Can you work these out from the model? Positions are in its coordinate system, mm. Round coordinates to 2 decimals unless told otherwise and drop trailing zeros. Loops run counter-clockwise (first coordinate to the right, second up) from the corner with the lowest first, then second, coordinate; pieces in that order, holes last.
(1) I want a section at B-B on x = 148.75. Write out the boundary of the cut face in (y, z), plus the area to 3 significant figures.
(2) I want a section at A-A on z = 51. Write out the boundary of the cut face in (x, y).
(3) Thinking about a two-plate mould opening in Z: for faces 1 (the face through (89, 0, 59)), 2 (the face through (176.99, 0.74, 17.85)), 3 (the face through (89.34, 0.76, 32.24)), 4 (the face through (176.99, 0.74, 102.15)), which applies, released by +Z, released by -Z, zero draft, split by the parting line, or undercut?
(4) I want a section at C-C on y = 1.2. Give the number of separate pieces and of enclosed holes in the cut face, plus the area to 3 significant figures.
(5) If I drill on line 1 along X through (y, z) = (0.3, 60); line 2 along Z through (x, y) = (148.75, 0.65); line 3 along X through (y, z) = (0.35, 31.25), over which ranges is the centre line in solid material (lowest first)?
(6) I want a section at D-D on x = 129. Write out the boundary of the cut face in (y, z).
from build123d import *

# Parameters (mm, degrees)
SKETCH1_W           = 180
SKETCH1_H           = 120
BOSS_EXTRUDE1_DEPTH = 1.5
SKETCH2_R           = 2.15
CUT_EXTRUDE1_DEPTH  = 217.33827678
SKETCH3_W           = 180
SKETCH3_H           = 15
CUT_EXTRUDE2_DEPTH  = 217.33827678
FILLET1_R           = 10


with BuildPart() as part:
    # Sketch1 → Boss-Extrude1 (new body)
    with BuildSketch(Plane(origin=(0, 0, 0), x_dir=(1, 0, 0), z_dir=(0, 1, 0))):
        with Locations((90, -60)):
            Rectangle(SKETCH1_W, SKETCH1_H)
    extrude(amount=BOSS_EXTRUDE1_DEPTH)

    # Sketch2 → Cut-Extrude1 (cut, through all)
    with BuildSketch(Plane(origin=(0, 1.5, 0), x_dir=(1, 0, 0), z_dir=(0, 1, 0))):
        with Locations(Location((120, -51, 0), (0, 0, 270))):
            Circle(SKETCH2_R)
        with Locations(Location((120, -69, 0), (0, 0, 270))):
            Circle(SKETCH2_R)
        with Locations(Location((129, -60, 0), (0, 0, 270))):
            Circle(SKETCH2_R)
        with Locations(Location((111, -60, 0), (0, 0, 270))):
            Circle(SKETCH2_R)
        with Locations(Location((78, -51, 0), (0, 0, 270))):
            Circle(SKETCH2_R)
        with Locations(Location((62, -51, 0), (0, 0, 270))):
            Circle(SKETCH2_R)
        with Locations(Location((62, -69, 0), (0, 0, 270))):
            Circle(SKETCH2_R)
        with Locations(Location((78, -69, 0), (0, 0, 270))):
            Circle(SKETCH2_R)
        with Locations(Location((148.75, -31.25, 0), (0, 0, 270))):
            Circle(SKETCH2_R)
        with Locations(Location((91.25, -31.25, 0), (0, 0, 270))):
            Circle(SKETCH2_R)
        with Locations(Location((91.25, -88.75, 0), (0, 0, 270))):
            Circle(SKETCH2_R)
        with Locations(Location((148.75, -88.75, 0), (0, 0, 270))):
            Circle(SKETCH2_R)
    extrude(amount=-CUT_EXTRUDE1_DEPTH, mode=Mode.SUBTRACT)

    # Sketch3 → Cut-Extrude2 (cut, through all)
    with BuildSketch(Plane(origin=(0, 1.5, 0), x_dir=(1, 0, 0), z_dir=(0, 1, 0))):
        with Locations((90, -7.5)):
            Rectangle(SKETCH3_W, SKETCH3_H)
        with Locations((90, -112.5)):
            Rectangle(SKETCH3_W, SKETCH3_H)
    extrude(amount=-CUT_EXTRUDE2_DEPTH, mode=Mode.SUBTRACT)

    # Fillet1
    fillet1_edges = [part.edges().sort_by_distance(p)[0] for p in [
        (0, 0.75, 15),
        (180, 0.75, 15),
        (0, 0.75, 105),
        (180, 0.75, 105),
    ]]
    fillet(fillet1_edges, radius=FILLET1_R)


solid = part.part
Filled sheet:
1. outline: (0, 15) - (1.5, 15) - (1.5, 29.1) - (0, 29.1) - close; (0, 33.4) - (1.5, 33.4) - (1.5, 86.6) - (0, 86.6) - close; (0, 90.9) - (1.5, 90.9) - (1.5, 105) - (0, 105) - close
1. area: 122 mm2
2. outline: (0, 0) - (59.85, 0) - (59.85, 1.5) - (0, 1.5) - close; (64.15, 0) - (75.85, 0) - (75.85, 1.5) - (64.15, 1.5) - close; (80.15, 0) - (117.85, 0) - (117.85, 1.5) - (80.15, 1.5) - close; (122.15, 0) - (180, 0) - (180, 1.5) - (122.15, 1.5) - close
3. face 1: zero draft
3. face 2: released by -Z
3. face 3: undercut
3. face 4: released by +Z
4. separate pieces: 1
4. enclosed holes: 12
4. area: 15,900 mm2
5. line 1: x = 0 to 108.85, 113.15 to 126.85, 131.15 to 180
5. line 2: z = 15 to 29.1, 33.4 to 86.6, 90.9 to 105
5. line 3: x = 0 to 89.1, 93.4 to 146.6, 150.9 to 180
6. outline: (0, 15) - (1.5, 15) - (1.5, 57.85) - (0, 57.85) - close; (0, 62.15) - (1.5, 62.15) - (1.5, 105) - (0, 105) - close
